from build123d import *

# Parameters (mm, degrees)
F0_W     = 603.25
F0_H     = 1016
F1_DEPTH = 279.4
F2_T     = -19.05
F3_W     = 565.15
F3_H     = 19.05
F4_DEPTH = 260.35


with BuildPart() as f1:
    # F0 (on Front) → F1 (new body)
    with BuildSketch(Plane.XZ):
        with Locations((301.625, 508)):
            Rectangle(F0_W, F0_H)
    extrude(amount=F1_DEPTH)

    # F2
    f2_openings = [f1.faces().sort_by_distance(p)[0] for p in [
        (301.625, -279.4, 508),
    ]]
    offset(amount=F2_T, openings=f2_openings)

    # F3 (on face) → F4 (join)
    with BuildSketch(Plane.XZ.offset(19.05)):
        with Locations((301.625, 733.425)):
            Rectangle(F3_W, F3_H)
        with Locations((301.625, 479.425)):
            Rectangle(F3_W, F3_H)
        with Locations((301.625, 225.425)):
            Rectangle(F3_W, F3_H)
    extrude(amount=F4_DEPTH)


solid = f1.part
Read the model definition and answer for the solid it produces. Units are mm, in the model's axes. A direction names the side the tool comes from. Round coordinates to 2 decimals unless told otherwise and drop trailing zeros. Write each loop counter-clockwise with the first axis right and the second up, starting at its lowest first coordinate (ties: lowest second). Pieces come first, ordered by that corner, then holes. Notation, with made-up numbers: M -18.75,79.5 L 35.25,79.5 A19 cw 35.25,105.5 Z; hole C -33.75,-15 d4. An arc over 180 degrees is marked long. Use a Markdown table: item, result.
1) For a pull along Z with two mould halves and no side action, classify faces 1 (the flat face through (298, -147, 996.95)), 2 (the flat face through (297, -138, 0)), 3 (the flat face through (0, -138, 501)) as pulls with the +Z half, pulls with the -Z half, needs draft (parallel to the pull), parting line crosses it, or undercut.
Answers follow:
| item | result |
|---|---|
| face 1 | undercut |
| face 2 | pulls with the -Z half |
| face 3 | needs draft |
2) The part is cut by section C-C (z = 174.5). Write down the section's boundary in (x, y), plus the area to 3 significant figures.
Answers follow:
| item | result |
|---|---|
| outline | M 0,-279.4 L 19.05,-279.4 L 19.05,-19.05 L 584.2,-19.05 L 584.2,-279.4 L 603.25,-279.4 L 603.25,0 L 0,0 Z |
| area | 21,400 mm2 |
3) A flat-ended cylindrical pin translates along its axis: pin 1 (1 mm diameter, centred on x = 316.5, z = 505.5, fed in from -Y). Find the tip coordinate at first contact, or state that the pin passes through.
Answers follow:
| item | result |
|---|---|
| pin 1 | stops at y = -19.05 |
4) The part is cut by section A-A (y = -94.5). Write down the section's boundary in (x, z), plus the area to 3 significant figures.
Answers follow:
| item | result |
|---|---|
| outline | M 0,0 L 603.25,0 L 603.25,1016 L 0,1016 Z; hole M 19.05,19.05 L 584.2,19.05 L 584.2,215.9 L 19.05,215.9 Z; hole M 19.05,234.95 L 584.2,234.95 L 584.2,469.9 L 19.05,469.9 Z; hole M 19.05,488.95 L 584.2,488.95 L 584.2,723.9 L 19.05,723.9 Z; hole M 19.05,742.95 L 584.2,742.95 L 584.2,996.95 L 19.05,996.95 Z |
| area | 92,500 mm2 |
5) A tool of negligible diameter and unlimited length cuts with its end or side. For faces 4 (the flat face through (298, -147, 488.95)), 5 (the flat face through (603.25, -138, 501)), from which of +Z, -Z, +X, -X, +Y, -Y can it reach the whole face along a straight path? Write none if from no direction.
Answers follow:
| item | result |
|---|---|
| face 4 | -Y |
| face 5 | +Z, -Z, +X, +Y, -Y |
6) The part is cut by section B-B (x = 538). Write down the section's boundary in (y, z), plus the area to 3 significant figures.
Answers follow:
| item | result |
|---|---|
| outline | M -279.4,0 L 0,0 L 0,1016 L -279.4,1016 L -279.4,996.95 L -19.05,996.95 L -19.05,742.95 L -279.4,742.95 L -279.4,723.9 L -19.05,723.9 L -19.05,488.95 L -279.4,488.95 L -279.4,469.9 L -19.05,469.9 L -19.05,234.95 L -279.4,234.95 L -279.4,215.9 L -19.05,215.9 L -19.05,19.05 L -279.4,19.05 Z |
| area | 44,200 mm2 |
7) Straight lines are drawn through the part: line 1 along Z through (x, y) = (109, -90); line 2 along X through (y, z) = (-135, 240); line 3 along Y through (x, z) = (178.5, 962). For each, find the intervals that lie inside material, in ascending order. Write a range as [from, to].
Answers follow:
| item | result |
|---|---|
| line 1 | z = [0, 19.05], [215.9, 234.95], [469.9, 488.95], [723.9, 742.95], [996.95, 1016] |
| line 2 | x = [0, 19.05], [584.2, 603.25] |
| line 3 | y = [-19.05, 0] |
